Autodesk Inventor part; units mm, degrees
ref_plane "作業平面1" through (0, 0, 0) normal (0, 0, 1) x (1, 0, 0)
ref_plane "作業平面2" through (0, 0, -8.3) normal (0, 0, -1) x (-1, 0, 0)
ref_plane "YZ Plane" through (0, 0, 0) normal (1, 0, 0) x (0, 1, 0)
ref_plane "作業平面1" through (0, 0, 0) normal (0, 0, 1) x (1, 0, 0)
ref_plane "作業平面2" through (0, 0, -8.3) normal (0, 0, -1) x (-1, 0, 0)
sketch "スケッチ1" plane through (0, 0, -8.3) normal (0, 0, -1) x (-1, 0, 0)
  circle A0 centre (0, -11.25) radius 6.5
  circle A1 centre (0, -11.25) radius 26
  line L0 (10, 12.75) -> (-10, 12.75)
  line L1 (11, -1.75) -> (-11, -1.75)
  line L2 (-13, -3.75) -> (-13, -18.75)
  line L3 (-11, -20.75) -> (11, -20.75)
  line L4 (13, -18.75) -> (13, -3.75)
  line L5 (13, -1.75) -> (-13, -20.75) construction
  line L6 (-13, -1.75) -> (13, -20.75) construction
  arc A2 (11, -20.75) -> (13, -18.75) centre (11, -18.75) ccw
  arc A3 (13, -3.75) -> (11, -1.75) centre (11, -3.75) ccw
  arc A4 (-11, -1.75) -> (-13, -3.75) centre (-11, -3.75) ccw
  arc A5 (-13, -18.75) -> (-11, -20.75) centre (-11, -18.75) ccw
  circle A6 centre (8, 8.2) radius 2.425
  circle A7 centre (-8, 8.2) radius 2.425
  circle A8 centre (8, 8.2) radius 1.875
  circle A9 centre (-8, 8.2) radius 1.875
  point P0 (0, 0)
  dimension "d0" = 52
  dimension "d1" = 20
  dimension "d2" = 26
  dimension "d3" = 19
  dimension "d4" = 2
  dimension "d7" = 3.75
extrude "押し出し1" add sketch "スケッチ1" along normal blind 1.5 contours A1 L0 | A6 | A7 picked at (-0.9365, -26.1993)
sketch "スケッチ2" plane through (0, 0, -8.3) normal (0, 0, 1) x (1, 0, 0)
  circle A0 centre (0, -11.25) radius 24
  arc A1 (-10, 12.75) -> (10, 12.75) centre (0, -11.25) ccw
  arc A2 (-13, 7.1144) -> (13, 7.1144) centre (0, -11.25) ccw
  line L0 (-13, 7.1144) -> (-13, 8.9242)
  line L1 (13, 7.1144) -> (13, 8.9242)
  point P0 (0, 0)
  point P1 (13, 8.0193)
  dimension "d8" = 48
  dimension "d9" = 1.5
  dimension "d10" = 26
extrude "押し出し2" add sketch "スケッチ2" against normal blind 8 contours A0 L0 A2 L1 picked at (18.6222, -25.3282)
properties part number "Mirror_Mount"
Verification items for the finished model (mm, model axes). A direction names the side the tool comes from. Round coordinates to 2 decimals unless told otherwise and drop trailing zeros. Loops run counter-clockwise (first coordinate to the right, second up) from the corner with the lowest first, then second, coordinate; pieces in that order, holes last. Notation, with made-up numbers: M -10.75,64.25 L 8.25,64.25 A24 cw 8.25,103.25 Z; hole C 47,81 d3. An arc over 180 degrees is marked long. Write each question's results on one line, items separated by ' | '.
1) Access from +Z, -Z, +X, -X, +Y, -Y to the whole of each face (thin tool, end or side, straight path). Record for faces 1 (the flat face through (7, -33, -16.3)), 2 (the flat face through (-13, 8, -13)), 3 (the cylindrical face through (-0.795, -33.736, -13.004)), 4 (the cylindrical face through (-12.43, -20.15, -9.04)).
Checks:
face 1: -Z, +X, -X, +Y, -Y | face 2: -Z, +Y | face 3: -Z | face 4: +Z, -Z
2) Section check C-C on z = -9. Record the boundary of the cut face in (x, y) (3 decimals).
Checks:
outline: M -10,12.75 A26 ccw long 10,12.75 Z; hole M -13,-18.75 A2 ccw -11,-20.75 L 11,-20.75 A2 ccw 13,-18.75 L 13,-3.75 A2 ccw 11,-1.75 L -11,-1.75 A2 ccw -13,-3.75 Z; hole C -8,8.2 d3.75; hole C 8,8.2 d3.75
3) Section check D-D on y = 8.2. Record the boundary of the cut face in (x, z) (1 decimal), then the cut area to 3 significant figures.
Checks:
outline: M -17.3,-9.8 L -14.1,-9.8 L -14.1,-16.3 L -13,-16.3 L -13,-9.8 L -9.9,-9.8 L -9.9,-8.3 L -17.3,-8.3 Z; M -6.1,-9.8 L 6.1,-9.8 L 6.1,-8.3 L -6.1,-8.3 Z; M 9.9,-9.8 L 13,-9.8 L 13,-16.3 L 14.1,-16.3 L 14.1,-9.8 L 17.3,-9.8 L 17.3,-8.3 L 9.9,-8.3 Z | area: 54.3 mm2
4) Section check B-B on y = -11.25. Record the boundary of the cut face in (x, z).
Checks:
outline: M -26,-9.8 L -24,-9.8 L -24,-16.3 L -22.5,-16.3 L -22.5,-9.8 L -13,-9.8 L -13,-8.3 L -26,-8.3 Z; M 13,-9.8 L 22.5,-9.8 L 22.5,-16.3 L 24,-16.3 L 24,-9.8 L 26,-9.8 L 26,-8.3 L 13,-8.3 Z
5) Gauge pin test, flat ends, axial feed: P1, Ø1, axis at x = -15, z = -9.5, coming from the -Y side; P2, Ø1.2, axis at y = -14.5, z = -9, coming from the +X side; P3, Ø5, axis at x = 8, y = 8.2, coming from the -Z side. Record the tip position at first contact, or that the pin passes through.
Checks:
P1: stops at y = -32.83 | P2: stops at x = 25.86 | P3: stops at z = -9.8
6) Section check A-A on x = 0. Record the boundary of the cut face in (y, z).
Checks:
outline: M -37.25,-9.8 L -35.25,-9.8 L -35.25,-16.3 L -33.75,-16.3 L -33.75,-9.8 L -20.75,-9.8 L -20.75,-8.3 L -37.25,-8.3 Z; M -1.75,-9.8 L 12.75,-9.8 L 12.75,-8.3 L -1.75,-8.3 Z
7) Mould release check, pull along Y, two halves, no side actions. Record for faces 5 (the cylindrical face through (12.43, -2.35, -9.04)), 6 (the flat face through (0, 12.75, -9)), 7 (the flat face through (0, -1, -8.3)): released by +Y, released by -Y, zero draft, split by the parting line, or undercut.
Checks:
face 5: undercut | face 6: released by +Y | face 7: zero draft
8) Scan lines: L1, parallel to X at y = -11.25, z = -13.25; L2, parallel to Y at x = -8, z = -9.3 (3 decimals); L3, parallel to Z at x = 12, y = 6. Record each from-to range of solid material in increasing order. Write a range as from..to.
Checks:
L1: x = -24..-22.5, 22.5..24 | L2: y = -35.989..-20.75, -1.75..6.325, 10.075..12.75 | L3: z = -9.8..-8.3
